Build history of the part. All positions in model axes, mm. A direction names the side the tool comes from. Give positions to 0.01 mm unless a question says otherwise; leave off trailing zeros. Loops run counter-clockwise (first coordinate to the right, second up) from the corner with the lowest first, then second, coordinate; pieces in that order, holes last. Notation, with made-up numbers: (40.25, -6) -> (63.25, -6) arc R10 ccw to (63.25, 9) -> close; hole circle Ø7 at (24.25, 28). An arc over 180 degrees is marked (long way). Answer as a JSON object with one key per item and string values. Group by question number.
Q1. Tool access for faces 1 (the flat face through (157, 0, -34)), 2 (the flat face through (65.088, 7, -33)), 3 (the cylindrical face through (8.347, 4.696, -10.435)): list every direction of +Z, -Z, +X, -X, +Y, -Y with a clear straight run to the whole face (end or side of a thin tool).
Q2. Drop flat-ended pins along their axis: pin 1 (2 mm diameter, centred on x = 74.5, z = -24, fed in from +Y); pin 2 (1.5 mm diameter, centred on y = -2.5, z = -45.5, fed in from -X) (3 decimals); pin 3 (8 mm diameter, centred on x = 9.525, z = -12.7, fed in from -Y). Give the stop position or say it passes through.
Q3. Band-saw the part on D-D, the plane x = 109. Write the cut outline in (y, z) (3 decimals).
Q4. Two-plate mould, pull along X, no slides. Class faces 4 (the cylindrical face through (92.29, -3.78, -33.8)), 5 (the flat face through (91, -4, -66.675)), 6 (the flat face through (130.175, -3, -33)): pulls with the +X half, pulls with the -X half, needs draft (parallel to the pull), parting line crosses it, or undercut.
Q5. Wall check: probe 1 along X at (y, z) = (5.75, -12.7); probe 2 along X at (y, z) = (5, -64); probe 3 along X at (y, z) = (-5, -11.5) (3 decimals). Give the ranges that are in metal, low to high. Write a range as from..to.
Q6. Band-saw the part on A-A, the plane z = -12.7. Count the separate pieces of the cut face and the enclosed holes in it, plus the area to 3 significant figures.
from build123d import *

# Parameters (mm, degrees)
SKETCH1_W              = 184.15
SKETCH1_H              = 66.675
BOSS_EXTRUDE1_DEPTH    = 9.525
SKETCH4_W              = 76.2
SKETCH4_H              = 6.35
BOSS_EXTRUDE2_DEPTH    = 66.675
SKETCH5_W              = 53.975
SKETCH5_H              = 66.675
CUT_EXTRUDE1_DEPTH     = 9.525
F_10_CLEARANCE_HOLE1_D = 5.1054
SKETCH12_R             = 31.019294643
CUT_EXTRUDE3_DEPTH     = 197.080350239
FILLET8_R              = 5.08
FILLET9_R              = 5.08


with BuildPart() as part:
    # Sketch1 → Boss-Extrude1 (new body)
    with BuildSketch(Plane(origin=(0, 0, 0), x_dir=(1, 0, 0), z_dir=(0, 1, 0))):
        with Locations((92.075, 33.3375)):
            Rectangle(SKETCH1_W, SKETCH1_H)
    extrude(amount=BOSS_EXTRUDE1_DEPTH)

    # Sketch4 → Boss-Extrude2 (add)
    with BuildSketch(Plane.XY):
        with Locations((92.075, -3.175)):
            Rectangle(SKETCH4_W, SKETCH4_H)
    extrude(amount=-BOSS_EXTRUDE2_DEPTH)

    # Sketch5 → Cut-Extrude1 (cut)
    with BuildSketch(Plane(origin=(0, 9.525, 0), x_dir=(1, 0, 0), z_dir=(0, 1, 0))):
        with Locations((92.075, 33.3375)):
            Rectangle(SKETCH5_W, SKETCH5_H)
    extrude(amount=-CUT_EXTRUDE1_DEPTH, mode=Mode.SUBTRACT)

    # #10 Clearance Hole1 (through all)
    with Locations(Plane(origin=(0, 9.525, 0), x_dir=(1, 0, 0), z_dir=(0, 1, 0))):
        with Locations((9.525, 53.975), (9.525, 12.7), (60.325, 12.7), (60.325, 53.975), (123.825, 53.975), (123.849810746, 12.7), (174.625, 12.7), (174.625, 53.975)):
            Hole(F_10_CLEARANCE_HOLE1_D / 2)

    # Sketch12 → Cut-Extrude3 (cut, through all)
    with BuildSketch(Plane(origin=(0, 0, -66.675), x_dir=(-1, 0, 0), z_dir=(0, 0, -1))):
        with Locations((-92.075, 27.239371317)):
            Circle(SKETCH12_R)
    extrude(amount=-CUT_EXTRUDE3_DEPTH, mode=Mode.SUBTRACT)

    # Fillet8
    fillet8_edges = [part.edges().sort_by_distance(p)[0] for p in [
        (65.0875, 0, -33.3375),
    ]]
    fillet(fillet8_edges, radius=FILLET8_R)

    # Fillet9
    fillet9_edges = [part.edges().sort_by_distance(p)[0] for p in [
        (119.0625, 0, -33.3375),
    ]]
    fillet(fillet9_edges, radius=FILLET9_R)


solid = part.part
Worked answers:
{
 "1": {"face 1": "+Z, -Z, +X, -Y", "face 2": "+Z, -Z, +Y", "face 3": "+Y, -Y"},
 "2": {"pin 1": "y = 0", "pin 2": "x = 53.975", "pin 3": "y = 0"},
 "3": {"outline": "(-6.35, -66.675) -> (0, -66.675) -> (0, 0) -> (-6.35, 0) -> close"},
 "4": {"face 4": "undercut", "face 5": "needs draft", "face 6": "pulls with the +X half"},
 "5": {"probe 1": "0..6.97, 12.08..57.77, 62.88..65.09, 119.06..121.3, 126.4..172.07, 177.18..184.15", "probe 2": "0..65.09, 119.06..184.15", "probe 3": "53.975..58.072, 62.578..121.597, 126.103..130.175"},
 "6": {"separate pieces": "5", "enclosed holes": "0", "area": "1,400 mm2"}
}
